```python
from build123d import *

# Parameters (mm, degrees)
F0_W     = 210
F0_H     = 130
F0_W_2   = 193
F0_H_2   = 111
F1_DEPTH = 4
F0_W_3   = 179
F0_H_3   = 97
F2_DEPTH = 1.5


with BuildPart() as f1:
    # F0 (on Top) → F1 (new body)
    with BuildSketch(Plane.XY):
        with Locations((48.212263, 14.238792)):
            Rectangle(F0_W, F0_H)
        with Locations((48.212263, 14.238792)):
            Rectangle(F0_W_2, F0_H_2, mode=Mode.SUBTRACT)
    extrude(amount=F1_DEPTH)

    # F0 (on Top) → F2 (join)
    with BuildSketch(Plane.XY):
        with Locations((48.212263, 14.238792)):
            Rectangle(F0_W_2, F0_H_2)
        with Locations((48.212263, 14.238792)):
            Rectangle(F0_W_3, F0_H_3, mode=Mode.SUBTRACT)
    extrude(amount=F2_DEPTH)


solid = f1.part
```
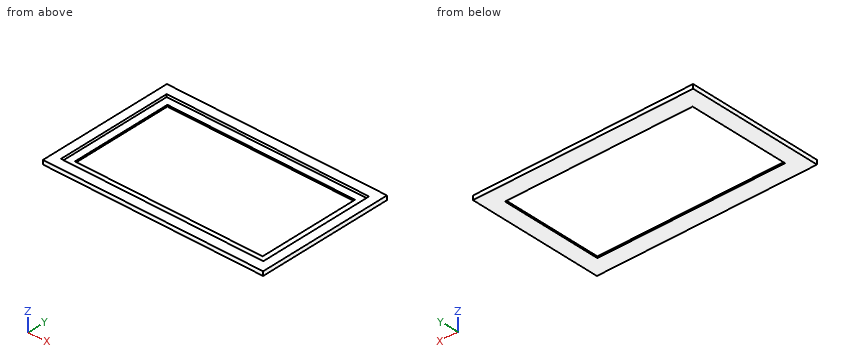
Design review of the part built by this model. Coordinates are the model's own, in mm. Coordinates: 2 decimals unless noted, no trailing zeros. Write each loop counter-clockwise with the first axis right and the second up, starting at its lowest first coordinate (ties: lowest second). Pieces come first, ordered by that corner, then holes.
1) Add section A-A (y = -20). Write out the cut boundary in (x, z), plus the area to 3 significant figures.
2) Add section B-B (z = 2.25). Write out the cut boundary in (x, y).
3) To check wall thickness, follow L1, parallel to X at y = -21, z = 2.3; L2, parallel to Y at x = 105, z = 0.4; L3, parallel to X at y = 33, z = 0.45. State the ranges of each line that lie inside material, in increasing order.
4) Add section C-C (x = 27.5). Write out the cut boundary in (y, z).
Check result:
1. outline: (-56.79, 0) - (-41.29, 0) - (-41.29, 1.5) - (-48.29, 1.5) - (-48.29, 4) - (-56.79, 4) - close; (137.71, 0) - (153.21, 0) - (153.21, 4) - (144.71, 4) - (144.71, 1.5) - (137.71, 1.5) - close
1. area: 89.0 mm2
2. outline: (-56.79, -50.76) - (153.21, -50.76) - (153.21, 79.24) - (-56.79, 79.24) - close; hole (-48.29, -41.26) - (144.71, -41.26) - (144.71, 69.74) - (-48.29, 69.74) - close
3. L1: x = -56.79 to -48.29, 144.71 to 153.21
3. L2: y = -50.76 to -34.26, 62.74 to 79.24
3. L3: x = -56.79 to -41.29, 137.71 to 153.21
4. outline: (-50.76, 0) - (-34.26, 0) - (-34.26, 1.5) - (-41.26, 1.5) - (-41.26, 4) - (-50.76, 4) - close; (62.74, 0) - (79.24, 0) - (79.24, 4) - (69.74, 4) - (69.74, 1.5) - (62.74, 1.5) - close
